from build123d import *

# Parameters (mm, degrees)
F0_W     = 80
F0_H     = 80
F0_W_2   = 50
F0_H_2   = 50
F1_DEPTH = 8
F2_DEPTH = 15
F4_DEPTH = 50
F5_R     = 5


with BuildPart() as f1:
    # F0 (on Top) → F1 (new body)
    with BuildSketch(Plane.XY):
        with Locations((-26.835108, 8.357681)):
            Rectangle(F0_W, F0_H)
        with Locations((-26.835108, 8.357681)):
            Rectangle(F0_W_2, F0_H_2, mode=Mode.SUBTRACT)
    extrude(amount=F1_DEPTH)

    # F0 (on Top) → F2 (join)
    with BuildSketch(Plane.XY):
        with Locations((-26.835108, 8.357681)):
            Rectangle(F0_W_2, F0_H_2)
    extrude(amount=F2_DEPTH)

    # F3 (on face) → F4 (cut, through all)
    with BuildSketch(Plane.XZ.offset(16.642319)):
        Polygon((-51.835108, 15), (-51.835108, 8), (-1.835108, 15), align=None)
    extrude(amount=-F4_DEPTH, mode=Mode.SUBTRACT)

    # F5
    f5_edges = [f1.edges().sort_by_distance(p)[0] for p in [
        (-26.835108, 48.357681, 8),
        (-66.835108, 8.357681, 8),
        (-26.835108, -31.642319, 8),
        (13.164892, 8.357681, 8),
    ]]
    fillet(f5_edges, radius=F5_R)


solid = f1.part
Model file for the job. Use its own axes, mm. A direction names the side the tool comes from. Give positions to 0.01 mm unless a question says otherwise; leave off trailing zeros. Loops run counter-clockwise (first coordinate to the right, second up) from the corner with the lowest first, then second, coordinate; pieces in that order, holes last.
Item 1: Drop flat-ended pins along their axis: P1, Ø7.5, axis at y = 2, z = 13, coming from the +X side; P2, Ø3.5, axis at x = -21, z = 11, coming from the -Y side; P3, Ø2, axis at x = -53.5, z = 5, coming from the -Y side; P4, Ø5, axis at x = -4, y = 22.5, coming from the -Z side. Give the stop position or say it passes through.
Check values:
P1: stops at x = -1.84
P2: stops at y = -16.64
P3: stops at y = -31.54
P4: stops at z = 0
Item 2: Slice it at A-A (y = 17). Write the cut outline in (x, z).
Check values:
outline: (-66.84, 0) - (13.16, 0) - (13.16, 3) arc R5 ccw to (8.16, 8) - (-1.84, 8) - (-1.84, 15) - (-51.84, 8) - (-61.84, 8) arc R5 ccw to (-66.84, 3) - close
Item 3: Drill centre lines: line 1 along Z through (x, y) = (3.5, 0); line 2 along Y through (x, z) = (-3, 8.5); line 3 along X through (y, z) = (34, 6.5). Where is each one in solid material? Low to high.
Check values:
line 1: z = 0 to 8
line 2: y = -16.64 to 33.36
line 3: x = -65.41 to 11.74
Item 4: Slice it at D-D (y = -25.5). Write the cut outline in (x, z), plus the area to 3 significant figures.
Check values:
outline: (-66.84, 0) - (13.16, 0) - (13.16, 3) arc R5 ccw to (8.16, 8) - (-61.84, 8) arc R5 ccw to (-66.84, 3) - close
area: 629 mm2
Item 5: Slice it at B-B (x = -49). Write the cut outline in (y, z).
Check values:
outline: (-31.64, 0) - (48.36, 0) - (48.36, 3) arc R5 ccw to (43.36, 8) - (33.36, 8) - (33.36, 8.4) - (-16.64, 8.4) - (-16.64, 8) - (-26.64, 8) arc R5 ccw to (-31.64, 3) - close
Item 6: Which spindle directions (+Z, -Z, +X, -X, +Y, -Y) get a long thin tool onto all of the face, cutting with end or side? Do faces 1 (the face through (-27, 9, 0)), 2 (the face through (-1.835, 8, 11)), 3 (the face through (-16, -16.642, 10)), 4 (the face through (-16, 33.358, 10)). Say none if no direction does.
Check values:
face 1: -Z, +X, -X, +Y, -Y
face 2: +Z, +X, +Y, -Y
face 3: +Z, +X, -X, -Y
face 4: +Z, +X, -X, +Y
Item 7: Slice it at C-C (z = 12.25). Write the cut outline in (x, y).
Check values:
outline: (-21.48, -16.64) - (-1.84, -16.64) - (-1.84, 33.36) - (-21.48, 33.36) - close
